from build123d import *

# Parameters (mm, degrees)
SKETCH1_R           = 34.29
BOSS_EXTRUDE1_DEPTH = 10.16
SKETCH2_R           = 33.02
CUT_EXTRUDE1_DEPTH  = 7.62
SKETCH3_R           = 3.81
BOSS_EXTRUDE2_DEPTH = 1.27
SKETCH4_R           = 1.27
BOSS_EXTRUDE3_DEPTH = 20.32
CUT_EXTRUDE3_REACH  = 55.082
CUT_EXTRUDE4_REACH  = 55.082
CUT_EXTRUDE5_REACH  = 56.165
SKETCH11_R          = 2.032


with BuildPart() as part:
    # Sketch1 → Boss-Extrude1 (new body)
    with BuildSketch(Plane(origin=(0, 0, 0), x_dir=(1, 0, 0), z_dir=(0, 1, 0))):
        with Locations(Location((0, 0, 0), (0, 0, 270))):
            Circle(SKETCH1_R)
    extrude(amount=BOSS_EXTRUDE1_DEPTH)

    # Sketch2 → Cut-Extrude1 (cut)
    with BuildSketch(Plane(origin=(0, 10.16, 0), x_dir=(1, 0, 0), z_dir=(0, 1, 0))):
        with Locations(Location((0, 0, 0), (0, 0, 270))):
            Circle(SKETCH2_R)
    extrude(amount=-CUT_EXTRUDE1_DEPTH, mode=Mode.SUBTRACT)

    # Sketch3 → Boss-Extrude2 (add)
    with BuildSketch(Plane(origin=(0, 2.54, 0), x_dir=(1, 0, 0), z_dir=(0, 1, 0))):
        with Locations(Location((0, -15.24, 0), (0, 0, 270))):
            Circle(SKETCH3_R)
        with Locations(Location((0, 15.24, 0), (0, 0, 270))):
            Circle(SKETCH3_R)
    extrude(amount=BOSS_EXTRUDE2_DEPTH)

    # Sketch4 → Boss-Extrude3 (add)
    with BuildSketch(Plane(origin=(0, 3.81, 0), x_dir=(1, 0, 0), z_dir=(0, 1, 0))):
        with Locations(Location((0, -15.24, 0), (0, 0, 270))):
            Circle(SKETCH4_R)
        with Locations(Location((0, 15.24, 0), (0, 0, 270))):
            Circle(SKETCH4_R)
    extrude(amount=BOSS_EXTRUDE3_DEPTH)

    # Sketch8 → Cut-Extrude3 (cut, up to next)
    with BuildSketch(Plane(origin=(0, 2.54, 0), x_dir=(1, 0, 0), z_dir=(0, 1, 0)), mode=Mode.PRIVATE) as cut_extrude3_sk1:
        with BuildLine():
            Line((3.683, 2.032), (-3.683, 2.032))
            ThreePointArc((-3.683, 2.032), (-4.581025612, 1.660025612), (-4.953, 0.762))
            Line((-4.953, 0.762), (-4.953, -0.762))
            ThreePointArc((-4.953, -0.762), (-4.581025612, -1.660025612), (-3.683, -2.032))
            Line((-3.683, -2.032), (3.683, -2.032))
            ThreePointArc((3.683, -2.032), (4.581025612, -1.660025612), (4.953, -0.762))
            Line((4.953, -0.762), (4.953, 0.762))
            ThreePointArc((4.953, 0.762), (4.581025612, 1.660025612), (3.683, 2.032))
        make_face()
    cut_extrude3_tool1 = extrude(cut_extrude3_sk1.sketch, amount=-CUT_EXTRUDE3_REACH, mode=Mode.PRIVATE) & part.part
    add(cut_extrude3_tool1.solids().sort_by_distance((0, 2.54, 0))[0], mode=Mode.SUBTRACT)

    # Sketch9 → Cut-Extrude4 (cut, up to next)
    with BuildSketch(Plane(origin=(0, 2.54, 0), x_dir=(1, 0, 0), z_dir=(0, 1, 0)), mode=Mode.PRIVATE) as cut_extrude4_sk1:
        with BuildLine():
            Line((-13.716, 0), (-11.176, 0))
            ThreePointArc((-11.176, 0), (-10.277974388, 0.371974388), (-9.906, 1.27))
            Line((-9.906, 1.27), (-9.906, 18.796))
            ThreePointArc((-9.906, 18.796), (-10.277974388, 19.694025612), (-11.176, 20.066))
            Line((-11.176, 20.066), (-13.716, 20.066))
            ThreePointArc((-13.716, 20.066), (-14.614025612, 19.694025612), (-14.986, 18.796))
            Line((-14.986, 18.796), (-14.986, 1.27))
            ThreePointArc((-14.986, 1.27), (-14.614025612, 0.371974388), (-13.716, 0))
        make_face()
    cut_extrude4_tool1 = extrude(cut_extrude4_sk1.sketch, amount=-CUT_EXTRUDE4_REACH, mode=Mode.PRIVATE) & part.part
    add(cut_extrude4_tool1.solids().sort_by_distance((-12.446, 2.54, -10.033))[0], mode=Mode.SUBTRACT)

    # Sketch11 → Cut-Extrude5 (cut, up to next)
    with BuildSketch(Plane.XZ, mode=Mode.PRIVATE) as cut_extrude5_sk1:
        with Locations(Location((15.875, 13.843, 0), (0, 0, 270))):
            Circle(SKETCH11_R)
    cut_extrude5_tool1 = extrude(cut_extrude5_sk1.sketch, amount=-CUT_EXTRUDE5_REACH, mode=Mode.PRIVATE) & part.part
    # Sketch11 → Cut-Extrude5 (cut, up to next)
    with BuildSketch(Plane.XZ, mode=Mode.PRIVATE) as cut_extrude5_sk2:
        with Locations(Location((-15.875, 13.843, 0), (0, 0, 270))):
            Circle(SKETCH11_R)
    cut_extrude5_tool2 = extrude(cut_extrude5_sk2.sketch, amount=-CUT_EXTRUDE5_REACH, mode=Mode.PRIVATE) & part.part
    # Sketch11 → Cut-Extrude5 (cut, up to next)
    with BuildSketch(Plane.XZ, mode=Mode.PRIVATE) as cut_extrude5_sk3:
        with Locations(Location((-15.875, -24.257, 0), (0, 0, 270))):
            Circle(SKETCH11_R)
    cut_extrude5_tool3 = extrude(cut_extrude5_sk3.sketch, amount=-CUT_EXTRUDE5_REACH, mode=Mode.PRIVATE) & part.part
    # Sketch11 → Cut-Extrude5 (cut, up to next)
    with BuildSketch(Plane.XZ, mode=Mode.PRIVATE) as cut_extrude5_sk4:
        with Locations(Location((15.875, -24.257, 0), (0, 0, 270))):
            Circle(SKETCH11_R)
    cut_extrude5_tool4 = extrude(cut_extrude5_sk4.sketch, amount=-CUT_EXTRUDE5_REACH, mode=Mode.PRIVATE) & part.part
    add(cut_extrude5_tool1.solids().sort_by_distance((15.875, 0, 13.843))[0], mode=Mode.SUBTRACT)
    add(cut_extrude5_tool2.solids().sort_by_distance((-15.875, 0, 13.843))[0], mode=Mode.SUBTRACT)
    add(cut_extrude5_tool3.solids().sort_by_distance((-15.875, 0, -24.257))[0], mode=Mode.SUBTRACT)
    add(cut_extrude5_tool4.solids().sort_by_distance((15.875, 0, -24.257))[0], mode=Mode.SUBTRACT)


solid = part.part
Geometry check sheet. Reference: the model listing, model coordinates, mm. A direction names the side the tool comes from. Give positions to 0.01 mm unless a question says otherwise; leave off trailing zeros. Write each loop counter-clockwise with the first axis right and the second up, starting at its lowest first coordinate (ties: lowest second). Pieces come first, ordered by that corner, then holes. Notation, with made-up numbers: M 29.5,64 L 88.5,64 A12 cw 88.5,83 Z; hole C -15.75,15 d2. An arc over 180 degrees is marked long. Answer as CSV lines item,"result". Start each with the question number.
Q1. Section check D-D, the plane z = 21.5. Record the cut outline in (x, y), then the cut area to 3 significant figures.
Q2. Material ranges on L1, parallel to Y at x = -2, z = 25; L2, parallel to Z at x = -0.5, y = 6.25; L3, parallel to Z at x = -16, y = 1.75, recorded low to high.
Q3. Section check B-B, the plane x = 0. Record the cut outline in (y, z), then the cut area to 3 significant figures.
Q4. Release check for a two-part mould opening along Z. For faces 1 (the face through (28, 10.16, -18)), 2 (the face through (-14.986, 1, -10)) record: pulls with the +Z half, pulls with the -Z half, needs draft (parallel to the pull), parting line crosses it, or undercut.
Q5. Section check C-C, the plane y = 8.5. Record the cut outline in (x, z), then the cut area to 3 significant figures.
Q6. Go/stop test with flat-tipped pins: pin 1 (6 mm diameter, centred on y = 8, z = -20, fed in from +X); pin 2 (1 mm diameter, centred on x = -7, z = 21, fed in from +Y); pin 3 (1.2 mm diameter, centred on y = 1.5, z = -0.5, fed in from -X); pin 4 (2.5 mm diameter, centred on x = -15.875, z = 13.843, fed in from +Y). Record where each tip stops, or that it passes through.
Q7. Section check A-A, the plane z = -10.5. Record the cut outline in (x, y), then the cut area to 3 significant figures.
Q8. Tool access check on faces 3 (the face through (1.144, 3.166, 18.874)), 4 (the face through (0, 24.13, -15)), 5 (the face through (-12, 1, 0)). Record the directions out of +Z, -Z, +X, -X, +Y, -Y that give a thin tool (end or side, any length) a straight path to the whole face; none if there is none.
Geometry says:
1,outline,"M -26.71,0 L 26.71,0 L 26.71,10.16 L 25.06,10.16 L 25.06,2.54 L -25.06,2.54 L -25.06,10.16 L -26.71,10.16 Z"
1,area,"161 mm^2"
2,L1,"0 to 2.54"
2,L2,"-34.29 to -33.02, -16.41 to -14.07, 14.07 to 16.41, 33.02 to 34.29"
2,L3,"-30.33 to -26.29, -22.23 to 11.81, 15.87 to 30.33"
3,outline,"M 0,-34.29 L 10.16,-34.29 L 10.16,-33.02 L 2.54,-33.02 L 2.54,-19.05 L 3.81,-19.05 L 3.81,-16.51 L 24.13,-16.51 L 24.13,-13.97 L 3.81,-13.97 L 3.81,-11.43 L 2.54,-11.43 L 2.54,-2.03 L 0,-2.03 Z; M 0,2.03 L 2.54,2.03 L 2.54,11.43 L 3.81,11.43 L 3.81,13.97 L 24.13,13.97 L 24.13,16.51 L 3.81,16.51 L 3.81,19.05 L 2.54,19.05 L 2.54,33.02 L 10.16,33.02 L 10.16,34.29 L 0,34.29 Z"
3,area,"306 mm^2"
4,face 1,"needs draft"
4,face 2,"undercut"
5,outline,"C 0,0 d68.58; C 0,-15.24 d2.54; C 0,15.24 d2.54; hole C 0,0 d66.04"
5,area,"279 mm^2"
6,pin 1,"x = 29.78"
6,pin 2,"y = 2.54"
6,pin 3,"x = -34.29"
6,pin 4,"through"
7,outline,"M -32.64,0 L -14.99,0 L -14.99,2.54 L -31.31,2.54 L -31.31,10.16 L -32.64,10.16 Z; M -9.91,0 L 32.64,0 L 32.64,10.16 L 31.31,10.16 L 31.31,2.54 L -9.91,2.54 Z"
7,area,"173 mm^2"
8,face 3,"+Y"
8,face 4,"+Z, -Z, +X, -X, +Y"
8,face 5,"+Y, -Y"
